```python
from build123d import *

# Parameters (mm, degrees)
BOSS_EXTRUDE1_DEPTH            = 1
F_1_5_1_5_DIAMETER_HOLE1_D     = 1.5
F_1_5_1_5_DIAMETER_HOLE1_DEPTH = 1
CUT_EXTRUDE2_DEPTH             = 2


with BuildPart() as part:
    # Sketch1 → Boss-Extrude1 (new body)
    with BuildSketch(Plane.XY):
        with BuildLine():
            Line((-9.623408959, -4.2), (-5.848076607, -4.2))
            ThreePointArc((-5.848076607, -4.2), (0, -7.2), (5.848076607, -4.2))
            Line((5.848076607, -4.2), (9.623408959, -4.2))
            ThreePointArc((9.623408959, -4.2), (0, -10.5), (-9.623408959, -4.2))
        make_face()
    extrude(amount=-BOSS_EXTRUDE1_DEPTH)

    # Ø1.5 (1.5) Diameter Hole1
    with Locations(Plane.XY):
        with Locations((0, -8.2), (-5.3, -6.256996084), (5.3, -6.256996084)):
            Hole(F_1_5_1_5_DIAMETER_HOLE1_D / 2, depth=F_1_5_1_5_DIAMETER_HOLE1_DEPTH)

    # Sketch2 → Cut-Extrude2 (cut, through all)
    with BuildSketch(Plane.XY):
        with BuildLine():
            Line((-7.903322086, -4.2), (-9.27823124, -4.915732403))
            ThreePointArc((-9.27823124, -4.915732403), (-9.457593181, -4.561132669), (-9.623408959, -4.2))
            Line((-9.623408959, -4.2), (-7.903322086, -4.2))
        make_face()
    cut_extrude2 = extrude(amount=-CUT_EXTRUDE2_DEPTH, mode=Mode.SUBTRACT)

    # Mirror1: Cut-Extrude2 across plane
    add(cut_extrude2.mirror(Plane(origin=(0, 0, 0), x_dir=(0, 0, 1), z_dir=(1, 0, 0))), mode=Mode.SUBTRACT)


solid = part.part
```
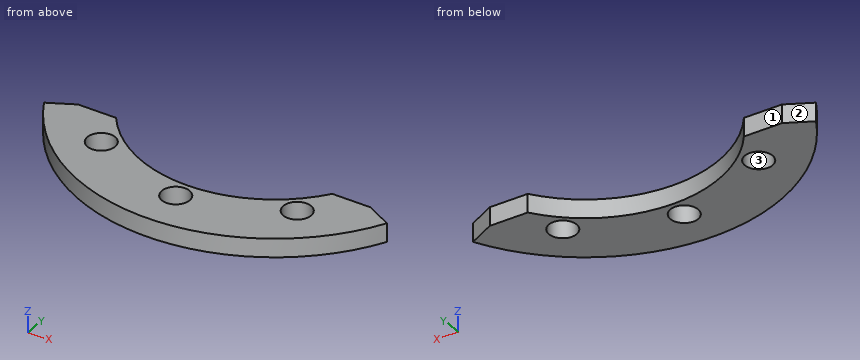
Verification items for the finished model (mm, model axes). Face numbers are marked on the shaded views. Coordinates: 2 decimals unless noted, no trailing zeros. Loops run counter-clockwise (first coordinate to the right, second up) from the corner with the lowest first, then second, coordinate; pieces in that order, holes last. Notation, with made-up numbers: (-19.75, 43.25) -> (13.25, 43.25) arc R30 cw to (13.25, 74.25) -> close; hole circle Ø7 at (5.5, 69). An arc over 180 degrees is marked (long way). Answer in a Markdown table with one row per item. Add a question column.
1. Draft check along X on the marked faces 1, 2 and 3. Enter one of: +X half, -X half, draft (parallel to the pull), parting line (faces both ways), or undercut.
2. Section check D-D, the plane x = 3.5. Enter the section's corners in (y, z), then the cut area to 3 significant figures.
3. Section check B-B, the plane y = -8.2. Enter the section's corners in (x, z), then the cut area to 3 significant figures.
4. Section check C-C, the plane z = -0.7. Enter the section's corners in (x, y).
5. Section check A-A, the plane x = 0. Enter the section's corners in (y, z).
6. Material ranges on probe 1 along X at (y, z) = (-6.25, -0.6); probe 2 along X at (y, z) = (-5.75, -0.9); probe 3 along Y at (x, z) = (-5.3, -0.5), recorded low to high. Write a range as [from, to].
Derived:
| question | item | result |
|---|---|---|
| 1 | face 1 | draft |
| 1 | face 2 | -X half |
| 1 | face 3 | undercut |
| 2 | outline | (-9.9, -1) -> (-6.29, -1) -> (-6.29, 0) -> (-9.9, 0) -> close |
| 2 | area | 3.61 mm² |
| 3 | outline | (-6.56, -1) -> (-0.75, -1) -> (-0.75, 0) -> (-6.56, 0) -> close; (0.75, -1) -> (6.56, -1) -> (6.56, 0) -> (0.75, 0) -> close |
| 3 | area | 11.6 mm² |
| 4 | outline | (-9.28, -4.92) arc R10.5 ccw to (9.28, -4.92) -> (7.9, -4.2) -> (5.85, -4.2) arc R7.2 cw to (-5.85, -4.2) -> (-7.9, -4.2) -> close; hole circle Ø1.5 at (-5.3, -6.26); hole circle Ø1.5 at (0, -8.2); hole circle Ø1.5 at (5.3, -6.26) |
| 5 | outline | (-10.5, -1) -> (-8.95, -1) -> (-8.95, 0) -> (-10.5, 0) -> close; (-7.45, -1) -> (-7.2, -1) -> (-7.2, 0) -> (-7.45, 0) -> close |
| 6 | probe 1 | x = [-8.44, -6.05], [-4.55, -3.57], [3.57, 4.55], [6.05, 8.44] |
| 6 | probe 2 | x = [-8.79, -5.85], [-4.75, -4.33], [4.33, 4.75], [5.85, 8.79] |
| 6 | probe 3 | y = [-9.06, -7.01], [-5.51, -4.87] |
